```python
from build123d import *

# Parameters (mm, degrees)
F0_R     = 76.2
F1_DEPTH = 25.4
F2_R     = 5.08
F4_DEPTH = 12.7


with BuildPart() as f1:
    # F0 (on Top) → F1 (new body)
    with BuildSketch(Plane.XY):
        Circle(F0_R)
    extrude(amount=F1_DEPTH)

    # F2
    f2_edges = [f1.edges().sort_by_distance(p)[0] for p in [
        (-76.2, 0, 25.4),
        (-76.2, 0, 0),
    ]]
    fillet(f2_edges, radius=F2_R)

    # F3 (on face) → F4 (join)
    with BuildSketch(Plane.XY.offset(25.4)):
        Polygon((-6.35, -10.998523), (6.35, -10.998523), (12.7, 0), (6.35, 10.998523), (-6.35, 10.998523), (-12.7, 0), align=None)
    extrude(amount=F4_DEPTH)


solid = f1.part
```
Can you work these out from the model? Positions are in its coordinate system, mm. A direction names the side the tool comes from. Coordinates: 2 decimals unless noted, no trailing zeros. Loops run counter-clockwise (first coordinate to the right, second up) from the corner with the lowest first, then second, coordinate; pieces in that order, holes last. Notation, with made-up numbers: (89.25, 87) -> (114.25, 87) arc R24 cw to (114.25, 125) -> close; hole circle Ø9 at (35, 40.5). An arc over 180 degrees is marked (long way). Answer as a JSON object with one key per item and string values.
1) For P1, Ø1, axis at y = -20.5, z = 17.5, coming from the -X side; P2, Ø1.5, axis at x = -29.5, z = 20.5, coming from the +Y side; P3, Ø1, axis at x = -31.5, y = -27.5, coming from the +Z side, each with a flat end and sliding along its axis, tell me the tip position at first contact or that it passes through.
Results:
{"P1": "stops at x = -73.53", "P2": "stops at y = 70.57", "P3": "stops at z = 25.4"}
2) Imagine slicing it at C-C (z = 9). Please give me the cut outline in (x, y), then the cut area to 3 significant figures.
Results:
{"outline": "circle Ø152.4 at (0, 0)", "area": "18,200 mm^2"}
3) Thinking about a two-plate mould opening in Z: for faces 1 (the face through (-1, 1, 0)), 2 (the face through (-1, -15, 25.4)), 3 (the face through (-9.57, -5.42, 31.66)), which applies, pulls with the +Z half, pulls with the -Z half, needs draft (parallel to the pull), parting line crosses it, or undercut?
Results:
{"face 1": "pulls with the -Z half", "face 2": "pulls with the +Z half", "face 3": "needs draft"}
4) Imagine slicing it at A-A (x = 0). Please give me the cut outline in (y, z), then the cut area to 3 significant figures.
Results:
{"outline": "(-76.2, 5.08) arc R5.08 ccw to (-71.12, 0) -> (71.12, 0) arc R5.08 ccw to (76.2, 5.08) -> (76.2, 20.32) arc R5.08 ccw to (71.12, 25.4) -> (11, 25.4) -> (11, 38.1) -> (-11, 38.1) -> (-11, 25.4) -> (-71.12, 25.4) arc R5.08 ccw to (-76.2, 20.32) -> close", "area": "4,130 mm^2"}
5) Imagine slicing it at B-B (z = 27.5). Please give me the cut outline in (x, y), then the cut area to 3 significant figures.
Results:
{"outline": "(-12.7, 0) -> (-6.35, -11) -> (6.35, -11) -> (12.7, 0) -> (6.35, 11) -> (-6.35, 11) -> close", "area": "419 mm^2"}
6) If I drill on line 1 (Z direction, x = -36, y = 51); line 2 (X direction, y = 1, z = 11.5); line 3 (Y direction, x = 13.5, z = 13.5), over which ranges is the centre line in solid material (lowest first)?
Results:
{"line 1": "z = 0 to 25.4", "line 2": "x = -76.19 to 76.19", "line 3": "y = -74.99 to 74.99"}
7) For faces 4 (the face through (0, -10.999, 32)), 5 (the face through (-9.48, 5.58, 31.66)), 6 (the face through (0, 10.999, 32)), 7 (the face through (9.48, -5.58, 31.66)), 8 (the face through (9.57, 5.42, 31.66)), which set-ups out of +Z, -Z, +X, -X, +Y, -Y let a thin tool reach every point of the face, with its end or its side?
Results:
{"face 4": "+Z, +X, -X, -Y", "face 5": "+Z, -X, +Y", "face 6": "+Z, +X, -X, +Y", "face 7": "+Z, +X, -Y", "face 8": "+Z, +X, +Y"}
